Build history of the part. All positions in model axes, mm. Face numbers are marked on the shaded views. A direction names the side the tool comes from. Round coordinates to 2 decimals unless told otherwise and drop trailing zeros. Write each loop counter-clockwise with the first axis right and the second up, starting at its lowest first coordinate (ties: lowest second). Pieces come first, ordered by that corner, then holes. Notation, with made-up numbers: (32.25, -20.5) -> (48.25, -20.5) arc R28 cw to (48.25, 12.5) -> close; hole circle Ø2 at (43, 66.5). An arc over 180 degrees is marked (long way). Answer in a Markdown table with one row per item. Add a question column.
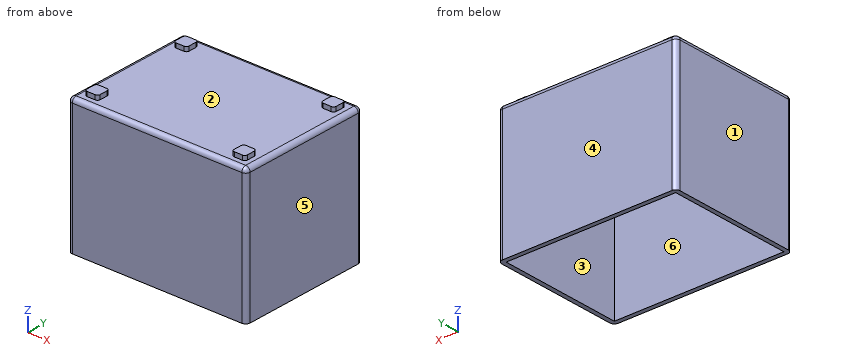
from build123d import *

# Parameters (mm, degrees)
SKETCH1_W           = 200
SKETCH1_H           = 150
BOSS_EXTRUDE1_DEPTH = 150
SKETCH2_W           = 190
SKETCH2_H           = 140
CUT_EXTRUDE1_DEPTH  = 145
SKETCH3_W           = 15
SKETCH3_H           = 15
BOSS_EXTRUDE3_DEPTH = 5
FILLET1_R           = 5
FILLET2_R           = 3


with BuildPart() as part:
    # Sketch1 → Boss-Extrude1 (new body)
    with BuildSketch(Plane.XY):
        with Locations((32.244318182, -44.957386364)):
            Rectangle(SKETCH1_W, SKETCH1_H)
    extrude(amount=BOSS_EXTRUDE1_DEPTH)

    # Sketch2 → Cut-Extrude1 (cut)
    with BuildSketch(Plane.XY):
        with Locations((32.244318182, -44.957386364)):
            Rectangle(SKETCH2_W, SKETCH2_H)
    extrude(amount=CUT_EXTRUDE1_DEPTH, mode=Mode.SUBTRACT)

    # Sketch3 → Boss-Extrude3 (add)
    with BuildSketch(Plane.XY.offset(150)):
        with Locations((-50.255681818, 12.542613636)):
            Rectangle(SKETCH3_W, SKETCH3_H)
        with Locations((114.744318182, 12.542613636)):
            Rectangle(SKETCH3_W, SKETCH3_H)
        with Locations((-50.255681818, -102.457386364)):
            Rectangle(SKETCH3_W, SKETCH3_H)
        with Locations((114.744318182, -102.457386364)):
            Rectangle(SKETCH3_W, SKETCH3_H)
    extrude(amount=BOSS_EXTRUDE3_DEPTH)

    # Fillet1
    fillet1_edges = [part.edges().sort_by_distance(p)[0] for p in [
        (132.244318182, -44.957386364, 150),
        (32.244318182, 30.042613636, 150),
        (-67.755681818, -44.957386364, 150),
        (-67.755681818, 30.042613636, 75),
        (132.244318182, 30.042613636, 75),
        (132.244318182, -119.957386364, 75),
        (-67.755681818, -119.957386364, 75),
        (32.244318182, -119.957386364, 150),
    ]]
    fillet(fillet1_edges, radius=FILLET1_R)

    # Fillet2
    fillet2_edges = [part.edges().sort_by_distance(p)[0] for p in [
        (-42.755681818, 5.042613636, 152.5),
        (-42.755681818, 20.042613636, 152.5),
        (-57.755681818, 20.042613636, 152.5),
        (-57.755681818, 5.042613636, 152.5),
        (122.244318182, 20.042613636, 152.5),
        (107.244318182, 20.042613636, 152.5),
        (107.244318182, 5.042613636, 152.5),
        (122.244318182, 5.042613636, 152.5),
        (-57.755681818, -94.957386364, 152.5),
        (-57.755681818, -109.957386364, 152.5),
        (-42.755681818, -109.957386364, 152.5),
        (-42.755681818, -94.957386364, 152.5),
        (122.244318182, -109.957386364, 152.5),
        (122.244318182, -94.957386364, 152.5),
        (107.244318182, -94.957386364, 152.5),
        (107.244318182, -109.957386364, 152.5),
    ]]
    fillet(fillet2_edges, radius=FILLET2_R)


solid = part.part
(1) Saw through at B-B (z = 37.5). List the corners of the cut face in (x, y), plus the area to 3 significant figures.
(2) Saw through at D-D (x = 113.5). List the corners of the cut face in (y, z), plus the area to 3 significant figures.
(3) Saw through at A-A (x = -7). List the corners of the cut face in (y, z), plus the area to 3 significant figures.
(4) Which spindle directions (+Z, -Z, +X, -X, +Y, -Y) get a long thin tool onto all of the face, cutting with end or side? Do the marked faces 1, 2 and 3. Say none if no direction does.
(5) Mould opens along Y. For the marked faces 4, 5 and 6 say: pulls with the +Y half, pulls with the -Y half, needs draft (parallel to the pull), parting line crosses it, or undercut.
(6) Probe line 1 along Y through (x, z) = (1, 120); line 2 along X through (y, z) = (-57, 70); line 3 along Z through (x, y) = (59, -19). List the from-to ranges inside material, lowest first.
(7) Saw through at C-C (y = -63.5). List the corners of the cut face in (x, z), plus the area to 3 significant figures.
(8) Drop flat-ended pins along their axis: P1, Ø1.5, axis at y = -101, z = 152, coming from the +X side; P2, Ø2.5, axis at y = -104.5, z = 152, coming from the -X side; P3, Ø5.5, axis at x = -51.5, z = 151.5, coming from the +Y side. Give the stop position or say it passes through.
Answer sheet:
| question | item | result |
|---|---|---|
| 1 | outline | (-67.76, -114.96) arc R5 ccw to (-62.76, -119.96) -> (127.24, -119.96) arc R5 ccw to (132.24, -114.96) -> (132.24, 25.04) arc R5 ccw to (127.24, 30.04) -> (-62.76, 30.04) arc R5 ccw to (-67.76, 25.04) -> close; hole (-62.76, -114.96) -> (127.24, -114.96) -> (127.24, 25.04) -> (-62.76, 25.04) -> close |
| 1 | area | 3,380 mm² |
| 2 | outline | (-119.96, 0) -> (-114.96, 0) -> (-114.96, 145) -> (25.04, 145) -> (25.04, 0) -> (30.04, 0) -> (30.04, 145) arc R5 ccw to (25.04, 150) -> (20.04, 150) -> (20.04, 155) -> (5.04, 155) -> (5.04, 150) -> (-94.96, 150) -> (-94.96, 155) -> (-109.96, 155) -> (-109.96, 150) -> (-114.96, 150) arc R5 ccw to (-119.96, 145) -> close |
| 2 | area | 2,340 mm² |
| 3 | outline | (-119.96, 0) -> (-114.96, 0) -> (-114.96, 145) -> (25.04, 145) -> (25.04, 0) -> (30.04, 0) -> (30.04, 145) arc R5 ccw to (25.04, 150) -> (-114.96, 150) arc R5 ccw to (-119.96, 145) -> close |
| 3 | area | 2,190 mm² |
| 4 | face 1 | +Z, -Z, -X, +Y, -Y |
| 4 | face 2 | +Z |
| 4 | face 3 | -Z |
| 5 | face 4 | pulls with the +Y half |
| 5 | face 5 | needs draft |
| 5 | face 6 | undercut |
| 6 | line 1 | y = -119.96 to -114.96, 25.04 to 30.04 |
| 6 | line 2 | x = -67.76 to -62.76, 127.24 to 132.24 |
| 6 | line 3 | z = 145 to 150 |
| 7 | outline | (-67.76, 0) -> (-62.76, 0) -> (-62.76, 145) -> (127.24, 145) -> (127.24, 0) -> (132.24, 0) -> (132.24, 145) arc R5 ccw to (127.24, 150) -> (-62.76, 150) arc R5 ccw to (-67.76, 145) -> close |
| 7 | area | 2,440 mm² |
| 8 | P1 | stops at x = 122.24 |
| 8 | P2 | stops at x = -57.76 |
| 8 | P3 | stops at y = 28.35 |
